Geometry: final body of the model. Coordinates: model frame, mm. A direction names the side the tool comes from. Give positions to 0.01 mm unless a question says otherwise; leave off trailing zeros. Loops run counter-clockwise (first coordinate to the right, second up) from the corner with the lowest first, then second, coordinate; pieces in that order, holes last.
Autodesk Inventor part; units mm, degrees
ref_plane "YZ Plane" through (0, 0, 0) normal (1, 0, 0) x (0, 1, 0)
ref_plane "XZ Plane" through (0, 0, 0) normal (0, 1, 0) x (-1, 0, 0)
ref_plane "XY Plane" through (0, 0, 0) normal (0, 0, 1) x (1, 0, 0)
sketch "Sketch1" plane through (0, 0, 0) normal (0, 1, 0) x (-1, 0, 0)
  line L0 (27.5, 18.707) -> (-27.5, 18.707)
  line L1 (-27.5, 18.707) -> (-27.5, -18.707)
  line L2 (-27.5, -18.707) -> (27.5, -18.707)
  line L3 (27.5, -18.707) -> (27.5, 18.707)
  line L4 (27.5, 18.707) -> (-27.5, -18.707) construction
  line L5 (-27.5, 18.707) -> (27.5, -18.707) construction
  point P0 (0, 0)
  dimension "d0" = 37.414
  dimension "d1" = 55
extrude "Extrusion1" add sketch "Sketch1" along normal blind 30.404
sketch "Sketch2" plane through (0, 30.404, 0) normal (0, 1, 0) x (1, 0, 0)
  line L0 (-26.5, -17.707) -> (26.5, -17.707)
  line L1 (26.5, -17.707) -> (26.5, 17.707)
  line L2 (26.5, 17.707) -> (-26.5, 17.707)
  line L3 (-26.5, 17.707) -> (-26.5, -17.707)
  line L4 (-26.5, -17.707) -> (26.5, 17.707) construction
  line L5 (26.5, -17.707) -> (-26.5, 17.707) construction
  point P0 (0, 0)
  dimension "d4" = 35.414
  dimension "d5" = 53
extrude "Extrusion2" cut sketch "Sketch2" against normal blind 29.404
sketch "Sketch6" plane through (0, 0, 0) normal (0, -1, 0) x (1, 0, 0)
  line L0 (175, 175) -> (-175, 175)
  line L1 (-175, 175) -> (-175, -175)
  line L2 (-175, -175) -> (175, -175)
  line L3 (175, -175) -> (175, 175)
  line L4 (175, 175) -> (-175, -175) construction
  line L5 (-175, 175) -> (175, -175) construction
  point P0 (0, 0)
  dimension "d19" = 350
  dimension "d20" = 350
extrude "Extrusion4" add sketch "Sketch6" along normal blind 2
sketch "Sketch7" plane through (0, -2, 0) normal (0, -1, 0) x (1, 0, 0)
  line L0 (39.5, 39.5) -> (-39.5, 39.5)
  line L1 (-39.5, 39.5) -> (-39.5, -39.5)
  line L2 (-39.5, -39.5) -> (39.5, -39.5)
  line L3 (39.5, -39.5) -> (39.5, 39.5)
  line L4 (39.5, 39.5) -> (-39.5, -39.5) construction
  line L5 (-39.5, 39.5) -> (39.5, -39.5) construction
  point P0 (0, 0)
  dimension "d23" = 79
  dimension "d24" = 79
extrude "Extrusion5" add sketch "Sketch7" along normal blind 11
sketch "Sketch8" plane through (0, -2, 0) normal (0, -1, 0) x (1, 0, 0)
  line L0 (2.3, -49) -> (-2.2, -49)
  line L1 (-2.2, -49) -> (-2.2, -44.5)
  line L2 (-2.2, -44.5) -> (2.3, -44.5)
  line L3 (2.3, -44.5) -> (2.3, -49)
  line L4 (2.3, -49) -> (-2.2, -44.5) construction
  line L5 (-2.2, -49) -> (2.3, -44.5) construction
  line L6 (-39.5, -39.5) -> (39.5, -39.5)
  line L7 (-175, 175) -> (-175, -175)
  point P0 (0, 0)
  point P1 (0.05, -46.75)
  dimension "d27" = 5
  dimension "d28" = 4.5
  dimension "d29" = 4.5
  dimension "d30" = 172.8
extrude "Extrusion6" add sketch "Sketch8" along normal blind 11
mirror "Mirror1" about plane through (0, 0, 0) normal (0, 0, 1) of "Extrusion6"
sketch "Sketch9" plane through (0, -2, 0) normal (0, -1, 0) x (1, 0, 0)
  line L0 (49, -2.3) -> (44.5, -2.3)
  line L1 (44.5, -2.3) -> (44.5, 2.2)
  line L2 (44.5, 2.2) -> (49, 2.2)
  line L3 (49, 2.2) -> (49, -2.3)
  line L4 (49, -2.3) -> (44.5, 2.2) construction
  line L5 (44.5, -2.3) -> (49, 2.2) construction
  line L6 (39.5, -39.5) -> (39.5, 39.5)
  line L7 (175, 175) -> (-175, 175)
  point P0 (0, 0)
  point P1 (46.75, -0.05)
  dimension "d33" = 5
  dimension "d34" = 4.5
  dimension "d35" = 4.5
  dimension "d36" = 172.8
extrude "Extrusion7" add sketch "Sketch9" along normal blind 11
mirror "Mirror2" about plane through (0, 0, 0) normal (1, 0, 0) of "Extrusion7"
sketch "Sketch10" plane through (0, -2, 0) normal (0, -1, 0) x (1, 0, 0)
  line L0 (49, 2.2) -> (49, -2.3)
  line L1 (49, -2.3) -> (49, -53.869)
  line L2 (2.3, -49) -> (58.6283, -49)
  line L3 (49, -49) -> (44.5, -49)
  line L4 (44.5, -49) -> (44.5, -39.5)
  line L5 (44.5, -39.5) -> (49, -39.5)
  line L6 (49, -39.5) -> (49, -49)
  line L7 (44.5, -44.25) -> (39.5, -44.25)
  line L8 (39.5, -44.25) -> (39.5, -49)
  line L9 (39.5, -49) -> (44.5, -49)
  line L10 (44.5, -49) -> (44.5, -44.25)
  point P0 (0, 0)
  dimension "d39" = 9.5
  dimension "d40" = 4.5
  dimension "d41" = 5
  dimension "d42" = 4.75
extrude "Extrusion8" add sketch "Sketch10" along normal blind 11
mirror "Mirror3" about plane through (0, 0, 0) normal (0, 0, 1) of "Extrusion8"
mirror "Mirror4" about plane through (0, 0, 0) normal (1, 0, 0) of "Extrusion8", "Mirror3"
properties part number "Motor-support_chassis-fit_hold-wheels_spencermical_ENES100-OSV"
Q1. Section query C-C, the plane x = -66. Return loops of the section in (y, z).
Q2. Material intervals for probe 1 along X at (y, z) = (13, -13); probe 2 along Z at (x, y) = (-8, 5.5); probe 3 along Y at (x, z) = (-83, -52), sorted ascending.
Q3. Mould query, pull axis Z, two halves, no side actions, for faces 4 (the face through (-26.5, 16, 0)), 5 (the face through (45, -13, 45)), 6 (the face through (44, -7, 49)). Classes: +Z half, -Z half, draft (parallel to the pull), parting line (faces both ways), or undercut.
Q4. Pin query (flat end, axial travel): pin 1 Ø5.5 at (x, y) = (15.5, -8) entering from -Z; pin 2 Ø2 at (y, z) = (-10, -47) entering from -X; pin 3 Ø1.3 at (x, y) = (-0.5, -9.5) entering from -Z; pin 4 Ø1.5 at (y, z) = (2.5, 112.5) entering from -X. Return the tip coordinate at first contact, or that it passes through.
Q5. Reachability of faces 1 (the face through (-49, -7, -44)), 2 (the face through (49, -7, -44)), 3 (the face through (0, 15, 18.707)) from +Z, -Z, +X, -X, +Y, -Y: full face, straight path, thin tool, end or side. Return the list, or none.
Q6. Section query A-A, the plane y = 14.5. Return loops of the section in (x, z).
Q7. Section query D-D, the plane z = -121. Return loops of the section in (x, y).
Q8. Section query B-B, the plane z = -27.5. Return loops of the section in (x, y), and give its area (3 significant figures).
Resolved:
1. outline: (-2, -175) - (0, -175) - (0, 175) - (-2, 175) - close
2. probe 1: x = -27.5 to -26.5, 26.5 to 27.5
2. probe 2: z = -18.71 to -17.71, 17.71 to 18.71
2. probe 3: y = -2 to 0
3. face 4: undercut
3. face 5: draft
3. face 6: +Z half
4. pin 1: stops at z = -39.5
4. pin 2: stops at x = -49
4. pin 3: stops at z = -49
4. pin 4: passes through
5. face 1: +Z, -Z, -X, -Y
5. face 2: +Z, -Z, +X, -Y
5. face 3: +Z, +X, -X, +Y
6. outline: (-27.5, -18.71) - (27.5, -18.71) - (27.5, 18.71) - (-27.5, 18.71) - close; hole (-26.5, -17.71) - (26.5, -17.71) - (26.5, 17.71) - (-26.5, 17.71) - close
7. outline: (-175, -2) - (175, -2) - (175, 0) - (-175, 0) - close
8. outline: (-175, -2) - (-39.5, -2) - (-39.5, -13) - (39.5, -13) - (39.5, -2) - (175, -2) - (175, 0) - (-175, 0) - close
8. area: 1,570 mm2
